The listing builds one solid part. Answer for the finished solid, in the listing's coordinates (mm). A direction names the side the tool comes from. Round coordinates to 2 decimals unless told otherwise and drop trailing zeros. Loops run counter-clockwise (first coordinate to the right, second up) from the corner with the lowest first, then second, coordinate; pieces in that order, holes last. Notation, with made-up numbers: (84, 16.25) - (130, 16.25) arc R23 ccw to (130, 27.25) - close; hole circle Ø1 at (60.25, 45.25). An arc over 180 degrees is marked (long way). One line per item, written item: value.
```python
from build123d import *

# Parameters (mm, degrees)
CROQUIS1_W              = 120
CROQUIS1_H              = 50
SALIENTE_EXTRUIR1_DEPTH = 15
CROQUIS2_W              = 50
CROQUIS2_H              = 25
SALIENTE_EXTRUIR2_DEPTH = 60
REDONDEO5_RADIUS        = 25
REDONDEO5_LENGTH        = 25
REDONDEO6_RADIUS        = 25
REDONDEO6_LENGTH        = 15
CROQUIS3_R              = 15
CORTAR_EXTRUIR1_DEPTH   = 89.459030065
CROQUIS4_R              = 15
CORTAR_EXTRUIR2_DEPTH   = 100.247166206


with BuildPart() as part:
    # Croquis1 → Saliente-Extruir1 (new body)
    with BuildSketch(Plane(origin=(0, 0, 0), x_dir=(1, 0, 0), z_dir=(0, 1, 0))):
        Rectangle(CROQUIS1_W, CROQUIS1_H)
    extrude(amount=SALIENTE_EXTRUIR1_DEPTH)

    # Croquis2 → Saliente-Extruir2 (add)
    with BuildSketch(Plane(origin=(0, 15, 0), x_dir=(1, 0, 0), z_dir=(0, 1, 0))):
        with Locations((-35, 12.5)):
            Rectangle(CROQUIS2_W, CROQUIS2_H)
    extrude(amount=SALIENTE_EXTRUIR2_DEPTH)

    # Redondeo5: full round fillet: the end face becomes a half cylinder, R = half its width
    redondeo5_face = Plane((-35, 75, -12.5), x_dir=(0, 0, 1), z_dir=(0, 1, 0))  # on the end face: x along it, z out of the body
    redondeo5_slab = redondeo5_face.offset(-REDONDEO5_RADIUS / 2) * Box(REDONDEO5_LENGTH, 2 * REDONDEO5_RADIUS, REDONDEO5_RADIUS, mode=Mode.PRIVATE)  # the body's end, R deep
    redondeo5_round = Plane((-35, 50, -12.5), x_dir=(0, 1, 0), z_dir=(0, 0, 1)) * Cylinder(REDONDEO5_RADIUS, REDONDEO5_LENGTH, mode=Mode.PRIVATE)  # its axis R under the face
    add(redondeo5_slab - redondeo5_round, mode=Mode.SUBTRACT)

    # Redondeo6: full round fillet: the end face becomes a half cylinder, R = half its width
    redondeo6_face = Plane((60, 7.5, 0), x_dir=(0, -1, 0), z_dir=(1, 0, 0))  # on the end face: x along it, z out of the body
    redondeo6_slab = redondeo6_face.offset(-REDONDEO6_RADIUS / 2) * Box(REDONDEO6_LENGTH, 2 * REDONDEO6_RADIUS, REDONDEO6_RADIUS, mode=Mode.PRIVATE)  # the body's end, R deep
    redondeo6_round = Plane((35, 7.5, 0), x_dir=(1, 0, 0), z_dir=(0, -1, 0)) * Cylinder(REDONDEO6_RADIUS, REDONDEO6_LENGTH, mode=Mode.PRIVATE)  # its axis R under the face
    add(redondeo6_slab - redondeo6_round, mode=Mode.SUBTRACT)

    # Croquis3 → Cortar-Extruir1 (cut, through all)
    with BuildSketch(Plane(origin=(0, 15, 0), x_dir=(1, 0, 0), z_dir=(0, 1, 0))):
        with Locations(Location((35, 0, 0), (0, 0, 270))):
            Circle(CROQUIS3_R)
    extrude(amount=-CORTAR_EXTRUIR1_DEPTH, mode=Mode.SUBTRACT)

    # Croquis4 → Cortar-Extruir2 (cut, through all)
    with BuildSketch(Plane.XY):
        with Locations((-35, 50)):
            Circle(CROQUIS4_R)
    extrude(amount=-CORTAR_EXTRUIR2_DEPTH, mode=Mode.SUBTRACT)


solid = part.part
```
1) A cutting plane is placed at D-D on z = 9.5. Give the vertices of the cut face in (x, y), and give its area (3 significant figures).
Final values:
outline: (-60, 0) - (23.39, 0) - (23.39, 15) - (-60, 15) - close; (46.61, 0) - (58.12, 0) - (58.12, 15) - (46.61, 15) - close
area: 1,420 mm2
2) Each of these flat-tipped pins is pushed along its axis until it touches: pin 1 Ø12.5 at (y, z) = (40, -9.5) entering from +X; pin 2 Ø5 at (x, z) = (16.5, -2) entering from -Y; pin 3 Ø6 at (x, z) = (32, -16.5) entering from +Y; pin 4 Ø6 at (x, y) = (-48, 52.5) entering from +Z. Where does it stop, or does it pass through?
Final values:
pin 1: x = -10
pin 2: y = 0
pin 3: y = 15
pin 4: z = 0
3) For a pull along X with two mould halves and no side action, classify faces 1 (the flat face through (-60, 19, -5)), 2 (the cylindrical face through (-46.056, 60.138, -12.325)), 3 (the cylindrical face through (-34.45, 74.994, -12.325)), 4 (the flat face through (-24, 29, -25)) as released by +X, released by -X, zero draft, split by the parting line, or undercut.
Final values:
face 1: released by -X
face 2: undercut
face 3: split by the parting line
face 4: zero draft
4) Consider L1, parallel to X at y = 3, z = 0; L2, parallel to Y at x = 1, z = 6; L3, parallel to Z at x = -43.5, y = 34. Determine where each line is inside the solid, lowest interval first.
Final values:
L1: -60 to 20, 50 to 60
L2: 0 to 15
L3: -25 to 0
5) For faces 5 (the flat face through (-10, 32, -12)), 6 (the flat face through (-13, 7, 25)), 7 (the flat face through (-35, 31, 0)), determine the directions among +Z, -Z, +X, -X, +Y, -Y from which every point of the face is accessible in a straight line to the end or side of a thin tool.
Final values:
face 5: +Z, -Z, +X, +Y
face 6: +Z, +X, -X, +Y, -Y
face 7: +Z, +X, -X, +Y
6) A cutting plane is placed at B-B on z = -8. Give the vertices of the cut face in (x, y), and give its area (3 significant figures).
Final values:
outline: (-60, 0) - (22.31, 0) - (22.31, 15) - (-10, 15) - (-10, 50) arc R25 ccw to (-60, 50) - close; (47.69, 0) - (58.69, 0) - (58.69, 15) - (47.69, 15) - close; hole circle Ø30 at (-35, 50)
area: 3,420 mm2
7) A cutting plane is placed at C-C on y = 62. Give the vertices of the cut face in (x, z), and give its area (3 significant figures).
Final values:
outline: (-56.93, -25) - (-44, -25) - (-44, 0) - (-56.93, 0) - close; (-26, -25) - (-13.07, -25) - (-13.07, 0) - (-26, 0) - close
area: 647 mm2
8) A cutting plane is placed at A-A on x = -35. Give the vertices of the cut face in (y, z), and give its area (3 significant figures).
Final values:
outline: (0, -25) - (35, -25) - (35, 0) - (15, 0) - (15, 25) - (0, 25) - close; (65, -25) - (75, -25) - (75, 0) - (65, 0) - close
area: 1,500 mm2
